Design review of the part built by this model. Coordinates are the model's own, in mm. A direction names the side the tool comes from. Round coordinates to 2 decimals unless told otherwise and drop trailing zeros. Loops run counter-clockwise (first coordinate to the right, second up) from the corner with the lowest first, then second, coordinate; pieces in that order, holes last. Notation, with made-up numbers: (-15, -7) -> (31, -7) arc R5 cw to (31, -2) -> close; hole circle Ø8 at (72.25, 57.5). An arc over 180 degrees is marked (long way). Use a Markdown table: item, result. Add a question column.
from build123d import *

# Parameters (mm, degrees)
BOSS_EXTRUDE1_DEPTH = 76.2
FILLET2_R           = 3.81
SKETCH2_R           = 3.175
CUT_EXTRUDE1_DEPTH  = 76.2
SKETCH3_R           = 3.175
CUT_EXTRUDE2_DEPTH  = 76.2


with BuildPart() as part:
    # Sketch1 → Boss-Extrude1 (new body)
    with BuildSketch(Plane(origin=(0, 0, 0), x_dir=(0, 0, -1), z_dir=(1, 0, 0))):
        Polygon((0.026896594, 23.297964889), (-25.373103406, 23.297964889), (-25.373103406, -2.102035111), (-19.023103406, -2.102035111), (-19.023103406, 16.947964889), (0.026896594, 16.947964889), align=None)
    extrude(amount=BOSS_EXTRUDE1_DEPTH)

    # Fillet2
    fillet2_edges = [part.edges().sort_by_distance(p)[0] for p in [
        (38.1, 16.947964889, -0.026896594),
        (38.1, -2.102035111, 19.023103406),
    ]]
    fillet(fillet2_edges, radius=FILLET2_R)

    # Sketch2 → Cut-Extrude1 (cut)
    with BuildSketch(Plane(origin=(0, 23.297964889, 0), x_dir=(1, 0, 0), z_dir=(0, 1, 0))):
        with Locations(Location((9.525, -9.498103406, 0), (0, 0, 270))):
            Circle(SKETCH2_R)
        with Locations(Location((66.675, -9.498103406, 0), (0, 0, 270))):
            Circle(SKETCH2_R)
    extrude(amount=-CUT_EXTRUDE1_DEPTH, mode=Mode.SUBTRACT)

    # Sketch3 → Cut-Extrude2 (cut)
    with BuildSketch(Plane.XY.offset(25.373103406)):
        with Locations((25.4, 7.422964889)):
            Circle(SKETCH3_R)
        with Locations((50.8, 7.422964889)):
            Circle(SKETCH3_R)
    extrude(amount=-CUT_EXTRUDE2_DEPTH, mode=Mode.SUBTRACT)


solid = part.part
1. Consider section D-D on x = 10.5. State the section outline as (y, z) points, plus the area to 3 significant figures.
2. To check wall thickness, follow probe 1 along Y at (x, z) = (50.8, 23.75); probe 2 along Z at (x, y) = (49.5, 3.25); probe 3 along Z at (x, y) = (30.5, 20.25). State the ranges of each line that lie inside material, in increasing order. Write a range as from..to.
3. For faces 5 (the face through (53.733, 6.207, 22.243)), 6 (the face through (38, 16.948, 12)), list the 3-axis set-ups (+Z, -Z, +X, -X, +Y, -Y) from which the entire face can be reached by the end or side of a thin tool; tool diameter is ignored.
4. Consider section B-B on y = 5.25. State the section outline as (x, z) points.
5. Mouldability with a two-part tool opening along X and no side actions: class faces 1 (the face through (0, 19, 18)), 2 (the face through (28.333, 6.207, 22.243)), 3 (the face through (38, 9, 19.023)), 4 (the face through (11.671, 20.167, 7.158)) as +X half, -X half, draft (parallel to the pull), parting line (faces both ways), or undercut.
6. Insertion check: P1, Ø5, axis at x = 9.52, z = 9.5, coming from the +Y side; P2, Ø2, axis at x = 31.5, z = 10.5, coming from the -Y side; P3, Ø8.5, axis at x = 50.8, y = 7.42, coming from the -Z side; P4, Ø12, axis at y = 6, z = 18.5, coming from the +X side. Each pin has a flat end and moves straight along its axis. Give the tip position at first contact, or say it passes through.
7. Consider section C-C on x = 60. State the section outline as (y, z) points, plus the area to 3 significant figures.
8. Consider section A-A on x = 50.8. State the section outline as (y, z) points.
Verdict:
| question | item | result |
|---|---|---|
| 1 | outline | (-2.1, 22.83) arc R3.81 ccw to (1.71, 19.02) -> (16.95, 19.02) -> (16.95, 12.52) -> (23.3, 12.52) -> (23.3, 25.37) -> (-2.1, 25.37) -> close; (16.95, 3.78) arc R3.81 ccw to (20.76, -0.03) -> (23.3, -0.03) -> (23.3, 6.48) -> (16.95, 6.48) -> close |
| 1 | area | 238 mm² |
| 2 | probe 1 | y = -2.1..4.25, 10.6..23.3 |
| 2 | probe 2 | z = 19.02..25.37 |
| 2 | probe 3 | z = 0.01..25.37 |
| 3 | face 5 | +Z, -Z |
| 3 | face 6 | -Z, +X, -X, -Y |
| 4 | outline | (0, 19.02) -> (23.09, 19.02) -> (23.09, 25.37) -> (0, 25.37) -> close; (27.71, 19.02) -> (48.49, 19.02) -> (48.49, 25.37) -> (27.71, 25.37) -> close; (53.11, 19.02) -> (76.2, 19.02) -> (76.2, 25.37) -> (53.11, 25.37) -> close |
| 5 | face 1 | -X half |
| 5 | face 2 | undercut |
| 5 | face 3 | draft |
| 5 | face 4 | undercut |
| 6 | P1 | passes through |
| 6 | P2 | stops at y = 16.95 |
| 6 | P3 | stops at z = 19.02 |
| 6 | P4 | stops at x = 76.2 |
| 7 | outline | (-2.1, 22.83) arc R3.81 ccw to (1.71, 19.02) -> (16.95, 19.02) -> (16.95, 3.78) arc R3.81 ccw to (20.76, -0.03) -> (23.3, -0.03) -> (23.3, 25.37) -> (-2.1, 25.37) -> close |
| 7 | area | 276 mm² |
| 8 | outline | (-2.1, 22.83) arc R3.81 ccw to (1.71, 19.02) -> (4.25, 19.02) -> (4.25, 25.37) -> (-2.1, 25.37) -> close; (10.6, 19.02) -> (16.95, 19.02) -> (16.95, 3.78) arc R3.81 ccw to (20.76, -0.03) -> (23.3, -0.03) -> (23.3, 25.37) -> (10.6, 25.37) -> close |
